```python
from build123d import *

# Parameters (mm, degrees)
F1_DEPTH = 10
F3_DEPTH = 10.001
F4_DEPTH = 3


# Not quite as in the source:
# - a pattern or mirror of a feature is missing from the dataset's text; its kind, count and spacing are read off the source's solid


with BuildPart() as f1:
    # F0 (on Front) → F1 (new body)
    with BuildSketch(Plane.XZ):
        Polygon((0, -10), (0, -6.25), (-5.25, -6.25), (-5.25, 0), (-13.25, 0), (-13.25, -10), align=None)
        Polygon((5.25, -6.25), (0, -6.25), (0, -10), (13.25, -10), (13.25, 0), (5.25, 0), align=None)
    extrude(amount=F1_DEPTH)

    # F2 (on face) → F3 (cut, through all)
    with BuildSketch(Plane.XY):
        with BuildLine():
            ThreePointArc((-9.25, -3.3), (-10.452081528, -3.797918472), (-10.95, -5))
            Line((-10.95, -5), (-9.25, -5))
            Line((-9.25, -5), (-9.25, -3.3))
        make_face()
        with BuildLine():
            Line((-9.25, -3.3), (-9.25, -5))
            Line((-9.25, -5), (-7.55, -5))
            ThreePointArc((-7.55, -5), (-8.047918472, -3.797918472), (-9.25, -3.3))
        make_face()
        with BuildLine():
            Line((-7.55, -5), (-9.25, -5))
            Line((-9.25, -5), (-9.25, -6.7))
            ThreePointArc((-9.25, -6.7), (-8.047918472, -6.202081528), (-7.55, -5))
        make_face()
        with BuildLine():
            Line((-9.25, -5), (-10.95, -5))
            ThreePointArc((-10.95, -5), (-10.452081528, -6.202081528), (-9.25, -6.7))
            Line((-9.25, -6.7), (-9.25, -5))
        make_face()
    f3 = extrude(amount=-F3_DEPTH, mode=Mode.SUBTRACT)

    # F3_copies: F3 across plane
    add(f3.mirror(Plane(origin=(0, 0, 0), x_dir=(0, 0, 1), z_dir=(1, 0, 0))), mode=Mode.SUBTRACT)

    # F2 (on face) → F4 (cut)
    with BuildSketch(Plane.XY):
        with BuildLine():
            Line((-12.15, -3.3256842194), (-12.15, -5))
            Line((-12.15, -5), (-10.95, -5))
            ThreePointArc((-10.95, -5), (-10.452081528, -3.797918472), (-9.25, -3.3))
            Line((-9.25, -3.3), (-9.25, -1.6513684387))
            Line((-9.25, -1.6513684387), (-12.15, -3.3256842194))
        make_face()
        with BuildLine():
            Line((-10.95, -5), (-12.15, -5))
            Line((-12.15, -5), (-12.15, -6.6743157806))
            Line((-12.15, -6.6743157806), (-9.25, -8.3486315613))
            Line((-9.25, -8.3486315613), (-9.25, -6.7))
            ThreePointArc((-9.25, -6.7), (-10.452081528, -6.202081528), (-10.95, -5))
        make_face()
        with BuildLine():
            Line((-9.25, -1.6513684387), (-9.25, -3.3))
            ThreePointArc((-9.25, -3.3), (-8.047918472, -3.797918472), (-7.55, -5))
            Line((-7.55, -5), (-6.35, -5))
            Line((-6.35, -5), (-6.35, -3.3256842194))
            Line((-6.35, -3.3256842194), (-9.25, -1.6513684387))
        make_face()
        with BuildLine():
            ThreePointArc((-7.55, -5), (-8.047918472, -6.202081528), (-9.25, -6.7))
            Line((-9.25, -6.7), (-9.25, -8.3486315613))
            Line((-9.25, -8.3486315613), (-6.35, -6.6743157806))
            Line((-6.35, -6.6743157806), (-6.35, -5))
            Line((-6.35, -5), (-7.55, -5))
        make_face()
    f4 = extrude(amount=-F4_DEPTH, mode=Mode.SUBTRACT)

    # F4_copies: F4 across plane
    add(f4.mirror(Plane(origin=(0, 0, 0), x_dir=(0, 0, 1), z_dir=(1, 0, 0))), mode=Mode.SUBTRACT)


solid = f1.part
```
Verification items for the finished model (mm, model axes). A direction names the side the tool comes from. Coordinates: 2 decimals unless noted, no trailing zeros. Loops run counter-clockwise (first coordinate to the right, second up) from the corner with the lowest first, then second, coordinate; pieces in that order, holes last. Notation, with made-up numbers: (-31.75, 71.5) - (-26.75, 71.5) arc R15 ccw to (-26.75, 75.5) - close; hole circle Ø1 at (43.25, 13.5). An arc over 180 degrees is marked (long way). Return JSON: item names as keys, results as strings.
1. Thickness scan on L1, parallel to X at y = -8, z = -5; L2, parallel to X at y = -4.5, z = -7; L3, parallel to Z at x = -4, y = -8. Record the ranges inside material, lowest first.
Established:
{"L1": "x = -13.25 to -5.25, 5.25 to 13.25", "L2": "x = -13.25 to -10.87, -7.63 to 7.63, 10.87 to 13.25", "L3": "z = -10 to -6.25"}
2. Go/stop test with flat-tipped pins: pin 1 (1.7 mm diameter, centred on x = 10, y = -3.5, fed in from +Z); pin 2 (3 mm diameter, centred on x = 1, y = -4, fed in from +Z). Record where each tip stops, or that it passes through.
Established:
{"pin 1": "stops at z = -3", "pin 2": "stops at z = -6.25"}
3. Section check B-B, the plane y = -4.75. Record the boundary of the cut face in (x, z).
Established:
{"outline": "(-13.25, -10) - (-10.93, -10) - (-10.93, -3) - (-12.15, -3) - (-12.15, 0) - (-13.25, 0) - close; (-7.57, -10) - (7.57, -10) - (7.57, -3) - (6.35, -3) - (6.35, 0) - (5.25, 0) - (5.25, -6.25) - (-5.25, -6.25) - (-5.25, 0) - (-6.35, 0) - (-6.35, -3) - (-7.57, -3) - close; (10.93, -10) - (13.25, -10) - (13.25, 0) - (12.15, 0) - (12.15, -3) - (10.93, -3) - close"}
4. Tool access check on faces 4 (the flat face through (0, 0, -7)), 5 (the flat face through (-5.25, -5, -3)), 6 (the flat face through (-7.82, -7.523, -1.479)). Record the directions out of +Z, -Z, +X, -X, +Y, -Y that give a thin tool (end or side, any length) a straight path to the whole face; none if there is none.
Established:
{"face 4": "+Z, -Z, +X, -X, +Y", "face 5": "+Z, +Y, -Y", "face 6": "+Z"}
5. Section check D-D, the plane z = -2.25. Record the boundary of the cut face in (x, y), then the cut area to 3 significant figures.
Established:
{"outline": "(-13.25, -10) - (-5.25, -10) - (-5.25, 0) - (-13.25, 0) - close; (5.25, -10) - (13.25, -10) - (13.25, 0) - (5.25, 0) - close; hole (-12.15, -6.67) - (-9.25, -8.35) - (-6.35, -6.67) - (-6.35, -3.33) - (-9.25, -1.65) - (-12.15, -3.33) - close; hole (6.35, -6.67) - (9.25, -8.35) - (12.15, -6.67) - (12.15, -3.33) - (9.25, -1.65) - (6.35, -3.33) - close", "area": "102 mm2"}
6. Mould release check, pull along X, two halves, no side actions. Record for faces 1 (the flat face through (-7.78, -2.5, -1.48)), 2 (the flat face through (0, -10, -7)), 3 (the flat face through (13.25, -5, -5)): +X half, -X half, draft (parallel to the pull), parting line (faces both ways), or undercut.
Established:
{"face 1": "undercut", "face 2": "draft", "face 3": "+X half"}
7. Section check A-A, the plane z = -4. Record the boundary of the cut face in (x, y).
Established:
{"outline": "(-13.25, -10) - (-5.25, -10) - (-5.25, 0) - (-13.25, 0) - close; (5.25, -10) - (13.25, -10) - (13.25, 0) - (5.25, 0) - close; hole circle Ø3.4 at (-9.25, -5); hole circle Ø3.4 at (9.25, -5)"}
8. Section check C-C, the plane x = 9. Record the boundary of the cut face in (y, z).
Established:
{"outline": "(-10, -10) - (-6.68, -10) - (-6.68, -3) - (-8.2, -3) - (-8.2, 0) - (-10, 0) - close; (-3.32, -10) - (0, -10) - (0, 0) - (-1.8, 0) - (-1.8, -3) - (-3.32, -3) - close"}
